from build123d import *

# Parameters (mm, degrees)
SKETCH1_W                   = 259.8
SKETCH1_H                   = 349.8
BOSS_EXTRUDE1_DEPTH         = 6.35
F_1_2_CLEARANCE_HOLE1_D     = 13.09624
F_1_2_CLEARANCE_HOLE1_DEPTH = 22.352
F_1_2_CLEARANCE_HOLE1_TIP   = 3.934507437
M8_CLEARANCE_HOLE1_D        = 8.4
M8_CLEARANCE_HOLE1_DEPTH    = 76.2
M8_CLEARANCE_HOLE1_TIP      = 2.5236146


with BuildPart() as part:
    # Sketch1 → Boss-Extrude1 (new body)
    with BuildSketch(Plane.XY):
        with Locations((-129.9, 174.9)):
            Rectangle(SKETCH1_W, SKETCH1_H)
    extrude(amount=BOSS_EXTRUDE1_DEPTH)

    # 1/2 Clearance Hole1
    with Locations(Plane.XY.offset(6.35)):
        with Locations((-129.9, 174.9)):
            Hole(F_1_2_CLEARANCE_HOLE1_D / 2, depth=F_1_2_CLEARANCE_HOLE1_DEPTH)
            with Locations((0, 0, -(F_1_2_CLEARANCE_HOLE1_DEPTH + F_1_2_CLEARANCE_HOLE1_TIP / 2))):  # 118° drill point
                Cone(0, F_1_2_CLEARANCE_HOLE1_D / 2, F_1_2_CLEARANCE_HOLE1_TIP, mode=Mode.SUBTRACT)

    # M8 Clearance Hole1
    with Locations(Plane.XY.offset(6.35)):
        with Locations((-237.3, 327.3), (-22.5, 327.3), (-22.5, 22.5), (-237.3, 22.5)):
            Hole(M8_CLEARANCE_HOLE1_D / 2, depth=M8_CLEARANCE_HOLE1_DEPTH)
            with Locations((0, 0, -(M8_CLEARANCE_HOLE1_DEPTH + M8_CLEARANCE_HOLE1_TIP / 2))):  # 118° drill point
                Cone(0, M8_CLEARANCE_HOLE1_D / 2, M8_CLEARANCE_HOLE1_TIP, mode=Mode.SUBTRACT)


solid = part.part
Part model, mm, in its own coordinate system. Round coordinates to 2 decimals unless told otherwise and drop trailing zeros. Loops run counter-clockwise (first coordinate to the right, second up) from the corner with the lowest first, then second, coordinate; pieces in that order, holes last. Notation, with made-up numbers: (-34, 76.5) - (-30, 76.5) arc R25 cw to (-30, 110.5) - close; hole circle Ø8 at (-20.75, -8.75). An arc over 180 degrees is marked (long way). Answer as a JSON object with one key per item and string values.
Item 1: Pull direction X, two halves, no side cores. Call faces 1 (the face through (-161, 177, 6.35)), 2 (the face through (-239.56, 26.04, 3.13)): pulls with the +X half, pulls with the -X half, needs draft (parallel to the pull), parting line crosses it, or undercut.
Output:
{"face 1": "needs draft", "face 2": "undercut"}
Item 2: Pin check, flat tip, straight feed: pin 1 (6.5 mm diameter, centred on x = -237.3, y = 22.5, fed in from -Z). Stop position of the tip, or through.
Output:
{"pin 1": "through"}
Item 3: Wall check: L1, parallel to X at y = 327.3, z = 3.75; L2, parallel to Y at x = -237.3, z = 4; L3, parallel to X at y = 328, z = 1.75. Give the ranges that are in metal, low to high.
Output:
{"L1": "-259.8 to -241.5, -233.1 to -26.7, -18.3 to 0", "L2": "0 to 18.3, 26.7 to 323.1, 331.5 to 349.8", "L3": "-259.8 to -241.44, -233.16 to -26.64, -18.36 to 0"}
Item 4: Band-saw the part on B-B on x = -129.9. List the corners of the cut face in (y, z).
Output:
{"outline": "(0, 0) - (168.35, 0) - (168.35, 6.35) - (0, 6.35) - close; (181.45, 0) - (349.8, 0) - (349.8, 6.35) - (181.45, 6.35) - close"}
Item 5: Band-saw the part on A-A on y = 22.5. List the corners of the cut face in (x, z), plus the area to 3 significant figures.
Output:
{"outline": "(-259.8, 0) - (-241.5, 0) - (-241.5, 6.35) - (-259.8, 6.35) - close; (-233.1, 0) - (-26.7, 0) - (-26.7, 6.35) - (-233.1, 6.35) - close; (-18.3, 0) - (0, 0) - (0, 6.35) - (-18.3, 6.35) - close", "area": "1,540 mm2"}
